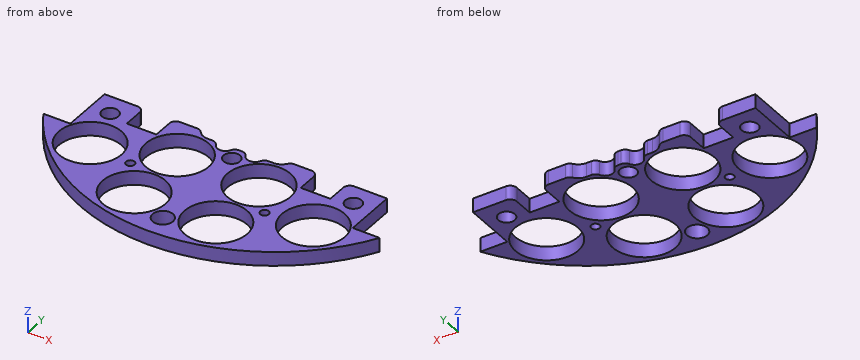
from build123d import *

# Parameters (mm, degrees)
SKETCH1_R                = 1.651
BOSS_EXTRUDE2_DEPTH      = 5.3975
SKETCH2_R                = 1.143
CUT_EXTRUDE1_DEPTH       = 6.3975
SKETCH3_R                = 12.1285
CUT_EXTRUDE2_DEPTH       = 6.3975
SKETCH4_W                = 28.562713242
SKETCH4_H                = 11.677503754
BOSS_EXTRUDE3_DEPTH      = 5.3975
SKETCH5_W                = 216.7214489
SKETCH5_H                = 130.569220634
CUT_EXTRUDE4_DEPTH       = 6.3975
SKETCH11_R               = 3.937
CUT_EXTRUDE11_DEPTH      = 6.3975
SKETCH12_W               = 11.43
SKETCH12_H               = 10.16
CUT_EXTRUDE12_DEPTH      = 6.3975
SKETCH16_R               = 12.192
CUT_EXTRUDE16_DEPTH      = 21.59
SKETCH57_R               = 1.651
CUT_EXTRUDE57_DEPTH      = 58.674
SKETCH58_R               = 3.175
CUT_EXTRUDE58_DEPTH      = 103.378
CUT_EXTRUDE58_DEPTH_BACK = 48.768
CUT_EXTRUDE15_DEPTH      = 21.59
FILLET1_R                = 2.54


with BuildPart() as part:
    # Sketch1 → Boss-Extrude2 (new body)
    with BuildSketch(Plane.XY):
        with BuildLine():
            Line((-64.964441474, 37.338), (-54.550441474, 37.338))
            Line((-54.550441474, 37.338), (-54.550441474, -37.338))
            Line((-54.550441474, -37.338), (-64.964441474, -37.338))
            ThreePointArc((-64.964441474, -37.338), (0, -74.93), (64.964441474, -37.338))
            Line((64.964441474, -37.338), (54.550441474, -37.338))
            Line((54.550441474, -37.338), (54.550441474, 37.338))
            Line((54.550441474, 37.338), (64.964441474, 37.338))
            ThreePointArc((64.964441474, 37.338), (0, 74.93), (-64.964441474, 37.338))
        make_face()
        with Locations((-46.482, 11.049)):
            Circle(SKETCH1_R, mode=Mode.SUBTRACT)
        with Locations((-21.083270032, 10.795)):
            Circle(SKETCH1_R, mode=Mode.SUBTRACT)
        with Locations((-21.083270032, -10.795)):
            Circle(SKETCH1_R, mode=Mode.SUBTRACT)
        with Locations((-46.482, -11.049)):
            Circle(SKETCH1_R, mode=Mode.SUBTRACT)
        with Locations((46.482, -11.049)):
            Circle(SKETCH1_R, mode=Mode.SUBTRACT)
        with Locations((21.083270032, -10.795)):
            Circle(SKETCH1_R, mode=Mode.SUBTRACT)
        with Locations((21.083270032, 10.795)):
            Circle(SKETCH1_R, mode=Mode.SUBTRACT)
        with Locations((46.482, 11.049)):
            Circle(SKETCH1_R, mode=Mode.SUBTRACT)
    extrude(amount=BOSS_EXTRUDE2_DEPTH)

    # Sketch2 → Cut-Extrude1 (cut, through all)
    with BuildSketch(Plane.XY.offset(5.3975)):
        with Locations((-6.731, 62.23)):
            Circle(SKETCH2_R)
        with Locations((6.731, 62.23)):
            Circle(SKETCH2_R)
    extrude(amount=-CUT_EXTRUDE1_DEPTH, mode=Mode.SUBTRACT)

    # Sketch3 → Cut-Extrude2 (cut, through all)
    with BuildSketch(Plane(origin=(0, 0, 0), x_dir=(-1, 0, 0), z_dir=(0, 0, -1))):
        with Locations((-15.777608989, -58.882838371)):
            Circle(SKETCH3_R)
        with Locations((15.777608989, -58.882838371)):
            Circle(SKETCH3_R)
        with Locations((-43.105229381, -43.105229381)):
            Circle(SKETCH3_R)
        with Locations((-43.105229381, 43.105229381)):
            Circle(SKETCH3_R)
        with Locations((43.105229381, 43.105229381)):
            Circle(SKETCH3_R)
        with Locations((43.105229381, -43.105229381)):
            Circle(SKETCH3_R)
    extrude(amount=-CUT_EXTRUDE2_DEPTH, mode=Mode.SUBTRACT)

    # Sketch4 → Boss-Extrude3 (add)
    with BuildSketch(Plane(origin=(0, 0, 0), x_dir=(-1, 0, 0), z_dir=(0, 0, -1))):
        with Locations((-1.488809975, 62.152540216)):
            Rectangle(SKETCH4_W, SKETCH4_H)
    extrude(amount=-BOSS_EXTRUDE3_DEPTH)

    # Sketch5 → Cut-Extrude4 (cut, through all)
    with BuildSketch(Plane(origin=(0, 0, 0), x_dir=(-1, 0, 0), z_dir=(0, 0, -1))):
        with Locations((23.316688373, 48.139610317)):
            Rectangle(SKETCH5_W, SKETCH5_H)
    extrude(amount=-CUT_EXTRUDE4_DEPTH, mode=Mode.SUBTRACT)

    # Sketch11 → Cut-Extrude11 (cut, through all)
    with BuildSketch(Plane(origin=(0, 0, 0), x_dir=(-1, 0, 0), z_dir=(0, 0, -1))):
        with Locations((0, -66.045)):
            Circle(SKETCH11_R)
    extrude(amount=-CUT_EXTRUDE11_DEPTH, mode=Mode.SUBTRACT)

    # Sketch12 → Cut-Extrude12 (cut, through all)
    with BuildSketch(Plane(origin=(0, 0, 0), x_dir=(-1, 0, 0), z_dir=(0, 0, -1))):
        with Locations((-33.595441474, -22.225)):
            Rectangle(SKETCH12_W, SKETCH12_H)
        with Locations((33.595441474, -22.225)):
            Rectangle(SKETCH12_W, SKETCH12_H)
    extrude(amount=-CUT_EXTRUDE12_DEPTH, mode=Mode.SUBTRACT)

    # Sketch16 → Cut-Extrude16 (cut)
    with BuildSketch(Plane(origin=(0, 0, 0), x_dir=(-1, 0, 0), z_dir=(0, 0, -1))):
        with Locations((15.777608989, -33.482838371)):
            Circle(SKETCH16_R)
        with Locations((-15.777608989, -33.482838371)):
            Circle(SKETCH16_R)
    extrude(amount=-CUT_EXTRUDE16_DEPTH, mode=Mode.SUBTRACT)

    # Sketch57 → Cut-Extrude57 (cut)
    with BuildSketch(Plane(origin=(0, 0, 0), x_dir=(-1, 0, 0), z_dir=(0, 0, -1))):
        with Locations((-25.937608989, -45.645229381)):
            Circle(SKETCH57_R)
        with Locations((25.937608989, -45.645229381)):
            Circle(SKETCH57_R)
    extrude(amount=-CUT_EXTRUDE57_DEPTH, mode=Mode.SUBTRACT)

    # Sketch58 → Cut-Extrude58 (cut, two sides)
    with BuildSketch(Plane(origin=(30.092005081, 4.08352975, 36.1315), x_dir=(-1, 0, 0), z_dir=(0, 0, -1))) as cut_extrude58_sk:
        with Locations((77.082005081, -29.48352975)):
            Circle(SKETCH58_R)
        with Locations((30.092005081, -29.48352975)):
            Circle(SKETCH58_R)
        with Locations((-16.897994919, -29.48352975)):
            Circle(SKETCH58_R)
    extrude(amount=CUT_EXTRUDE58_DEPTH, mode=Mode.SUBTRACT)
    extrude(cut_extrude58_sk.sketch, amount=-CUT_EXTRUDE58_DEPTH_BACK, mode=Mode.SUBTRACT)

    # Sketch15 → Cut-Extrude15 (cut)
    with BuildSketch(Plane(origin=(0, 0, 0), x_dir=(-1, 0, 0), z_dir=(0, 0, -1))):
        with BuildLine():
            Line((-12.7, -20.24), (-8.888991966, -20.24))
            ThreePointArc((-8.888991966, -20.24), (-5.715, -23.495), (-2.541008034, -20.24))
            Line((-2.541008034, -20.24), (2.541008034, -20.24))
            ThreePointArc((2.541008034, -20.24), (5.715, -23.495), (8.888991966, -20.24))
            Line((8.888991966, -20.24), (12.7, -20.24))
            ThreePointArc((12.7, -20.24), (16.235533906, -11.704466094), (7.7, -15.24))
            Line((7.7, -15.24), (-1.06, -15.24))
            ThreePointArc((-1.06, -15.24), (-4.010609847, -10.6792983), (-9.38, -11.501337137))
            ThreePointArc((-9.38, -11.501337137), (-17.374040774, -13.464234575), (-12.7, -20.24))
        make_face()
    extrude(amount=-CUT_EXTRUDE15_DEPTH, mode=Mode.SUBTRACT)

    # Fillet1
    fillet1_edges = [part.edges().sort_by_distance(p)[0] for p in [
        (39.310441474, -17.145, 2.69875),
        (27.880441474, -17.145, 2.69875),
        (-27.880441474, -17.145, 2.69875),
        (-39.310441474, -17.145, 2.69875),
        (-17.322875188, -17.145, 2.69875),
        (17.322875188, -17.145, 2.69875),
        (-8.888991966, -20.24, 2.69875),
        (-2.541008034, -20.24, 2.69875),
        (2.541008034, -20.24, 2.69875),
        (8.888991966, -20.24, 2.69875),
    ]]
    fillet(fillet1_edges, radius=FILLET1_R)


solid = part.part
The model under review builds one solid part; all positions refer to its coordinate system, in mm. Coordinates: 2 decimals unless noted, no trailing zeros. Loops run counter-clockwise (first coordinate to the right, second up) from the corner with the lowest first, then second, coordinate; pieces in that order, holes last. Notation, with made-up numbers: (-10.75, -6) -> (28.25, -6) arc R23 cw to (28.25, 7) -> close; hole circle Ø1 at (12.25, 61). An arc over 180 degrees is marked (long way). Use a Markdown table: item, result. Add a question column.
1. To check wall thickness, follow line 1 (Y direction, x = -15, z = 2.7); line 2 (X direction, y = -50.5, z = 4.2); line 3 (Y direction, x = -20, z = 5.2) (3 decimals). State the ranges of each line that lie inside material, in increasing order.
2. Add section A-A on y = -25.4. Give the number of separate pieces and of enclosed holes in the cut face, plus the area to 3 significant figures.
3. Add section B-B on x = -46. Write out the cut boundary in (y, z) (1 decimal), plus the area to 3 significant figures.
4. Add section D-D on y = -57. Write out the cut boundary in (x, z), plus the area to 3 significant figures.
5. Clearance check with flat-ended pins moving along their axes: pin 1 Ø2.5 at (y, z) = (-25, 3) entering from -X; pin 2 Ø2 at (x, y) = (-33, -51.5) entering from -Z; pin 3 Ø2.5 at (x, z) = (-36, 2.5) entering from +Y (3 decimals); pin 4 Ø1.5 at (x, z) = (12, 1.5) entering from +Y. State where each tip first meets the part, or that it passes through.
6. Add section C-C on y = -41.5. Write out the cut boundary in (x, z), plus the area to 3 significant figures.
Returned:
| question | item | result |
|---|---|---|
| 1 | line 1 | y = -73.41 to -70.99, -46.78 to -45.65, -21.32 to -19.68 |
| 1 | line 2 | x = -55.36 to -52.72, -33.49 to -24.54, -7.01 to 7.01, 24.54 to 33.49, 52.72 to 55.36 |
| 1 | line 3 | y = -72.212 to -70.253, -47.513 to -44.92, -22.045 to -17.145 |
| 2 | separate pieces | 8 |
| 2 | enclosed holes | 0 |
| 2 | area | 166 mm² |
| 3 | outline | (-59.1, 0) -> (-54.9, 0) -> (-54.9, 5.4) -> (-59.1, 5.4) -> close; (-31.3, 0) -> (-28.4, 0) -> (-28.4, 5.4) -> (-31.3, 5.4) -> close; (-22.4, 0) -> (-17.1, 0) -> (-17.1, 5.4) -> (-22.4, 5.4) -> close |
| 3 | area | 67.0 mm² |
| 4 | outline | (-48.64, 0) -> (-27.76, 0) -> (-27.76, 5.4) -> (-48.64, 5.4) -> close; (-3.8, 0) -> (3.8, 0) -> (3.8, 5.4) -> (-3.8, 5.4) -> close; (27.76, 0) -> (48.64, 0) -> (48.64, 5.4) -> (27.76, 5.4) -> close |
| 4 | area | 266 mm² |
| 5 | pin 1 | stops at x = -54.55 |
| 5 | pin 2 | stops at z = 0 |
| 5 | pin 3 | stops at y = -27.305 |
| 5 | pin 4 | stops at y = -20.24 |
| 6 | outline | (-62.39, 0) -> (-55.13, 0) -> (-55.13, 5.4) -> (-62.39, 5.4) -> close; (-31.08, 0) -> (-24.96, 0) -> (-24.96, 5.4) -> (-31.08, 5.4) -> close; (-6.59, 0) -> (6.59, 0) -> (6.59, 5.4) -> (-6.59, 5.4) -> close; (24.96, 0) -> (31.08, 0) -> (31.08, 5.4) -> (24.96, 5.4) -> close; (55.13, 0) -> (62.39, 0) -> (62.39, 5.4) -> (55.13, 5.4) -> close |
| 6 | area | 216 mm² |
